Could you check a few things on this model? Use its own coordinates, in mm. A direction names the side the tool comes from. Round coordinates to 2 decimals unless told otherwise and drop trailing zeros. Loops run counter-clockwise (first coordinate to the right, second up) from the corner with the lowest first, then second, coordinate; pieces in that order, holes last.
from build123d import *

# Parameters (mm, degrees)
SKETCH1_R                  = 2.794
SKETCH1_R_2                = 1.8415
BOSS_EXTRUDE1_DEPTH        = 3.2131
BOSS_EXTRUDE2_DEPTH        = 1.0922
M1_6_CLEARANCE_HOLE1_D     = 1.8
M1_6_CLEARANCE_HOLE1_DEPTH = 7.25
M1_6_CLEARANCE_HOLE1_TIP   = 0.540774557
SKETCH4_R                  = 1.651
CUT_EXTRUDE2_DEPTH         = 0.127
SKETCH5_W                  = 3
SKETCH5_H                  = 1
BOSS_EXTRUDE3_DEPTH        = 30
BOSS_EXTRUDE4_DEPTH        = 3
FILLET1_R                  = 0.5
RIB1_START                 = -0.5
RIB1_DEPTH                 = 1
RIB3_START                 = -0.5
RIB3_DEPTH                 = 1
BOSS_EXTRUDE8_DEPTH        = 1.5
FILLET2_R                  = 0.25


# Read off the part's stored shape, not the designer's step: Rib1, Rib3
with BuildPart() as part:
    # Sketch1 → Boss-Extrude1 (new body)
    with BuildSketch(Plane(origin=(0, 0, 0), x_dir=(1, 0, 0), z_dir=(0, 1, 0))):
        with Locations(Location((0, 0, 0), (0, 0, 270))):
            Circle(SKETCH1_R)
        with Locations(Location((0, 0, 0), (0, 0, 270))):
            Circle(SKETCH1_R_2, mode=Mode.SUBTRACT)
    extrude(amount=BOSS_EXTRUDE1_DEPTH)

    # Sketch2 → Boss-Extrude2 (add)
    with BuildSketch(Plane(origin=(0, 0, 0), x_dir=(1, 0, 0), z_dir=(0, 1, 0))):
        with BuildLine():
            Line((-1.5, 6.604), (-1.5, 2.357209367))
            ThreePointArc((-1.5, 2.357209367), (0, -2.794), (1.5, 2.357209367))
            Line((1.5, 2.357209367), (1.5, 6.604))
            Line((1.5, 6.604), (1.5, 13))
            Line((1.5, 13), (-1.5, 13))
            Line((-1.5, 13), (-1.5, 6.604))
        make_face()
    extrude(amount=BOSS_EXTRUDE2_DEPTH)

    # M1.6 Clearance Hole1
    with Locations(Plane(origin=(0, 1.0922, 0), x_dir=(1, 0, 0), z_dir=(0, 1, 0))):
        with Locations((0, 0)):
            Hole(M1_6_CLEARANCE_HOLE1_D / 2, depth=M1_6_CLEARANCE_HOLE1_DEPTH)
            with Locations((0, 0, -(M1_6_CLEARANCE_HOLE1_DEPTH + M1_6_CLEARANCE_HOLE1_TIP / 2))):  # 118° drill point
                Cone(0, M1_6_CLEARANCE_HOLE1_D / 2, M1_6_CLEARANCE_HOLE1_TIP, mode=Mode.SUBTRACT)

    # Sketch4 → Cut-Extrude2 (cut)
    with BuildSketch(Plane.XZ):
        with Locations(Location((0, 0, 0), (0, 0, 270))):
            Circle(SKETCH4_R)
    extrude(amount=-CUT_EXTRUDE2_DEPTH, mode=Mode.SUBTRACT)

    # Sketch5 → Boss-Extrude3 (add)
    with BuildSketch(Plane.XZ):
        with Locations((0, -12.5)):
            Rectangle(SKETCH5_W, SKETCH5_H)
    extrude(amount=-BOSS_EXTRUDE3_DEPTH)

    # Sketch6 → Boss-Extrude4 (add)
    with BuildSketch(Plane(origin=(1.5, 0, 0), x_dir=(0, 0, -1), z_dir=(1, 0, 0))):
        Polygon((22, 29), (12, 30), (12, 31.004987562), (22.099503719, 29.99503719), align=None)
    extrude(amount=-BOSS_EXTRUDE4_DEPTH)

    # Fillet1
    fillet1_edges = [part.edges().sort_by_distance(p)[0] for p in [
        (0, 0, -13),
        (0, 1.0922, -12),
        (0, 29, -22),
        (0, 31.004987562, -12),
        (0, 29.9, -13),
    ]]
    fillet(fillet1_edges, radius=FILLET1_R)

    # Rib1 outline → Rib1 (add)
    with BuildSketch(Plane(origin=(0, 0, 0), x_dir=(0, 0, -1), z_dir=(1, 0, 0)).offset(RIB1_START)):
        with BuildLine():
            Line((12, 1.5922), (12, 4.0922))
            Line((12, 4.0922), (7, 1.0922))
            Line((7, 1.0922), (11.5, 1.0922))
            ThreePointArc((11.5, 1.0922), (11.853553391, 1.238646609), (12, 1.5922))
        make_face()
    extrude(amount=RIB1_DEPTH)

    # Rib3 outline → Rib3 (add)
    with BuildSketch(Plane(origin=(0, 0, 0), x_dir=(0, 0, -1), z_dir=(1, 0, 0)).offset(RIB3_START)):
        with BuildLine():
            Line((13, 24.99503719), (18, 29.4))
            Line((18, 29.4), (13.54975186, 29.845024814))
            ThreePointArc((13.54975186, 29.845024814), (13.16449734, 29.718232486), (13, 29.347506219))
            Line((13, 29.347506219), (13, 24.99503719))
        make_face()
    extrude(amount=RIB3_DEPTH)

    # Sketch11 → Boss-Extrude8 (add, symmetric)
    with BuildSketch(Plane(origin=(0, 0, 0), x_dir=(0, 0, -1), z_dir=(1, 0, 0))):
        Polygon((2.357209367, 1.0922), (4.557209367, 1.0922), (2.794, 3.2131), (2.357209367, 3.2131), align=None)
    extrude(amount=BOSS_EXTRUDE8_DEPTH, both=True)

    # Fillet2
    fillet2_edges = [part.edges().sort_by_distance(p)[0] for p in [
        (-1.5, 1.60655, -2.357209367),
        (1.5, 1.60655, -2.357209367),
        (0, 3.2131, -2.794),
        (0, 1.0922, -4.557209367),
    ]]
    fillet(fillet2_edges, radius=FILLET2_R)


solid = part.part
Item 1: For faces 1 (the flat face through (0.5, 2, -11)), 2 (the flat face through (-0.007, 2.613, -9.535)), 3 (the flat face through (1, 1.092, -8)), 4 (the flat face through (0.5, 28, -14)), 5 (the flat face through (1.5, 14.4, -12.2)), which set-ups out of +Z, -Z, +X, -X, +Y, -Y let a thin tool reach every point of the face, with its end or its side?
Results list:
face 1: +X, +Y
face 2: +X, -X, +Y
face 3: +Y
face 4: +X, -Y
face 5: -Z, +X, +Y, -Y
Item 2: We'd pull the mould along X, two halves only. Please class faces 6 (the flat face through (-0.5, 28, -14)), 7 (the cylindrical face through (-0.86, 0.6, -0.27)), 8 (the flat face through (0, 0, -5)): released by +X, released by -X, zero draft, split by the parting line, or undercut.
Results list:
face 6: released by -X
face 7: undercut
face 8: zero draft
Item 3: If I drill on line 1 along Z through (x, y) = (0.8, 29); line 2 along Z through (x, y) = (2.1, 2.5); line 3 along Z through (x, y) = (0, 0.45), over which ranges is the centre line in solid material (lowest first)?
Results list:
line 1: z = -13 to -12
line 2: z = -1.84 to 1.84
line 3: z = -13 to -0.9, 0.9 to 2.79
Item 4: Will these pins go through, and if not, where does the flat tip stop? pin 1 (2.5 mm diameter, centred on x = 0, y = 13.5, fed in from -Z); pin 2 (2.5 mm diameter, centred on x = 0.5, z = -0.5, fed in from -Y); pin 3 (4 mm diameter, centred on y = 26.5, z = -15.5, fed in from -X); pin 4 (1.5 mm diameter, centred on y = 3, z = -10.5, fed in from +X).
Results list:
pin 1: stops at z = -13
pin 2: stops at y = 0
pin 3: stops at x = -0.5
pin 4: stops at x = 0.5
Item 5: If we section it at C-C, the plane y = 21: Please give me the cut outline in (x, z).
Results list:
outline: (-1.5, -13) - (1.5, -13) - (1.5, -12) - (-1.5, -12) - close
Item 6: If we section it at A-A, the plane z = 0: Please give me the cut outline in (x, y).
Results list:
outline: (-2.79, 0) - (-1.65, 0) - (-1.65, 0.13) - (-0.9, 0.13) - (-0.9, 1.09) - (-1.84, 1.09) - (-1.84, 3.21) - (-2.79, 3.21) - close; (0.9, 0.13) - (1.65, 0.13) - (1.65, 0) - (2.79, 0) - (2.79, 3.21) - (1.84, 3.21) - (1.84, 1.09) - (0.9, 1.09) - close
Item 7: If we section it at D-D, the plane z = -9: Please give me the cut outline in (x, y), then the cut area to 3 significant figures.
Results list:
outline: (-1.5, 0) - (1.5, 0) - (1.5, 1.09) - (0.5, 1.09) - (0.5, 2.29) - (-0.5, 2.29) - (-0.5, 1.09) - (-1.5, 1.09) - close
area: 4.48 mm2
